from build123d import *

# Parameters (mm, degrees)
F0_R     = 12.7
F1_DEPTH = 12.7
F2_R     = 3.302
F3_DEPTH = 12.7
F4_R     = 2.54
F5_DEPTH = 12.7


with BuildPart() as f1:
    # F0 (on Front) → F1 (new body)
    with BuildSketch(Plane.XZ):
        Circle(F0_R)
    extrude(amount=F1_DEPTH)

    # F2 (on face) → F3 (cut)
    with BuildSketch(Plane.XZ.offset(12.7)):
        Circle(F2_R)
    extrude(amount=-F3_DEPTH, mode=Mode.SUBTRACT)

    # F4 (on face) → F5 (join)
    with BuildSketch(Plane.XZ.offset(12.7)):
        with Locations((1.24495, 7.337332)):
            Circle(F4_R)
        with Locations((-6.593507, 3.451378)):
            Circle(F4_R)
        with Locations((-5.319961, -5.204263)):
            Circle(F4_R)
        with Locations((3.30559, -6.66779)):
            Circle(F4_R)
        with Locations((7.362928, 1.083342)):
            Circle(F4_R)
    extrude(amount=F5_DEPTH)


solid = f1.part
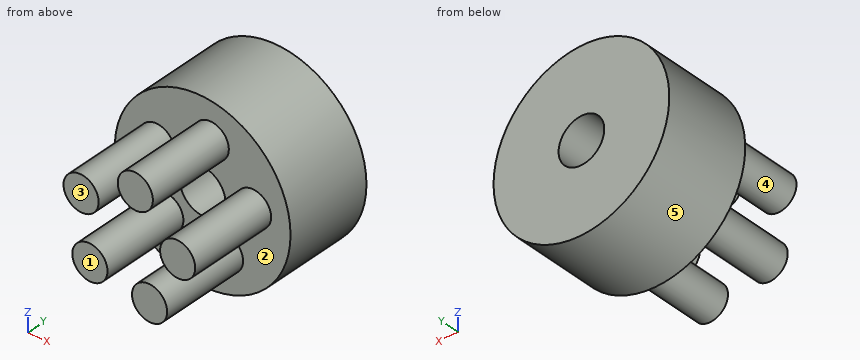
Could you check a few things on this model? Use its own coordinates, in mm. Face numbers are marked on the shaded views. A direction names the side the tool comes from. Coordinates: 2 decimals unless noted, no trailing zeros. Loops run counter-clockwise (first coordinate to the right, second up) from the corner with the lowest first, then second, coordinate; pieces in that order, holes last. Notation, with made-up numbers: (-32, 20) -> (-7, 20) arc R14 ccw to (-7, 27) -> close; hole circle Ø1 at (72.5, 50.5). An arc over 180 degrees is marked (long way). Answer in a Markdown table with one row per item.
(1) Imagine slicing it at A-A (x = 0). List the corners of the cut face in (y, z) for me, plus the area to 3 significant figures.
Results found:
| item | result |
|---|---|
| outline | (-25.4, 5.12) -> (-12.7, 5.12) -> (-12.7, 3.3) -> (0, 3.3) -> (0, 12.7) -> (-12.7, 12.7) -> (-12.7, 9.55) -> (-25.4, 9.55) -> close; (-12.7, -12.7) -> (0, -12.7) -> (0, -3.3) -> (-12.7, -3.3) -> close |
| area | 295 mm^2 |
(2) Imagine slicing it at D-D (y = -13.75). List the corners of the cut face in (x, z) for me, plus the area to 3 significant figures.
Results found:
| item | result |
|---|---|
| outline | circle Ø5.08 at (-6.59, 3.45); circle Ø5.08 at (-5.32, -5.2); circle Ø5.08 at (1.24, 7.34); circle Ø5.08 at (3.31, -6.67); circle Ø5.08 at (7.36, 1.08) |
| area | 101 mm^2 |
(3) Imagine slicing it at C-C (y = -10.5). List the corners of the cut face in (x, z) for me.
Results found:
| item | result |
|---|---|
| outline | circle Ø25.4 at (0, 0); hole circle Ø6.6 at (0, 0) |
(4) If I drill on probe 1 along Z at (x, y) = (0, -5.5); probe 2 along Y at (x, z) = (8, -4.75); probe 3 along X at (y, z) = (-19, 5), over which ranges is the centre line in solid material (lowest first)?
Results found:
| item | result |
|---|---|
| probe 1 | z = -12.7 to -3.3, 3.3 to 12.7 |
| probe 2 | y = -12.7 to 0 |
| probe 3 | x = -8.61 to -4.58, 0.25 to 2.24 |
(5) Thinking about a two-plate mould opening in Z: for the marked faces 3, 4 and 5, which applies, released by +Z, released by -Z, zero draft, split by the parting line, or undercut?
Results found:
| item | result |
|---|---|
| face 3 | zero draft |
| face 4 | undercut |
| face 5 | split by the parting line |
(6) Imagine slicing it at B-B (z = 0). List the corners of the cut face in (x, y) for me.
Results found:
| item | result |
|---|---|
| outline | (-12.7, -12.7) -> (-3.3, -12.7) -> (-3.3, 0) -> (-12.7, 0) -> close; (3.3, -12.7) -> (5.07, -12.7) -> (5.07, -25.4) -> (9.66, -25.4) -> (9.66, -12.7) -> (12.7, -12.7) -> (12.7, 0) -> (3.3, 0) -> close |
(7) Will these pins go through, and if not, where does the flat tip stop? pin 1 Ø5 at (x, y) = (3, -6.5) entering from -Z; pin 2 Ø10 at (y, z) = (-14, -7) entering from -X; pin 3 Ø1.5 at (y, z) = (-8.5, 8.5) entering from -X.
Results found:
| item | result |
|---|---|
| pin 1 | stops at z = -12.69 |
| pin 2 | stops at x = -12.51 |
| pin 3 | stops at x = -10.06 |
(8) For the marked faces 1 and 2, which set-ups out of +Z, -Z, +X, -X, +Y, -Y let a thin tool reach every point of the face, with its end or its side?
Results found:
| item | result |
|---|---|
| face 1 | +Z, -Z, +X, -X, -Y |
| face 2 | -Y |
